from build123d import *

# Parameters (mm, degrees)
F1_DEPTH = 63.5
F2_DEPTH = 63.5


with BuildPart() as f1:
    # F0 (on Front) → F1 (new body)
    with BuildSketch(Plane.XZ):
        Polygon((-177.549966, -85.353864), (-177.549966, -100.162064), (-156.467966, -100.162064), (-13.263665, 3.495336), (-29.975966, 3.495336), (-51.057966, 3.495336), (-51.057966, -11.312864), (-72.139966, -11.312864), (-72.139966, -26.121064), (-93.221966, -26.121064), (-93.221966, -40.929264), (-114.303966, -40.929264), (-114.303966, -55.737464), (-135.385966, -55.737464), (-135.385966, -70.545664), (-156.467966, -70.545664), (-156.467966, -85.353864), align=None)
        Polygon((-29.975966, 3.495336), (-13.263665, 3.495336), (33.524034, 3.495336), (33.524034, 18.303536), (-29.975966, 18.303536), align=None)
    extrude(amount=F1_DEPTH)

    # F0 (on Front) → F2 (join)
    with BuildSketch(Plane.XZ):
        Polygon((-156.467966, 93.080176), (-29.975966, 3.495336), (-29.975966, 18.303536), (-29.975966, 33.111736), (-51.057966, 33.111736), (-51.057966, 47.919936), (-72.139966, 47.919936), (-72.139966, 62.728136), (-93.221966, 62.728136), (-93.221966, 77.536336), (-114.303966, 77.536336), (-114.303966, 92.344536), (-135.385966, 92.344536), (-135.385966, 107.152736), (-156.467966, 107.152736), align=None)
        Polygon((-29.975966, 3.495336), (-13.263665, 3.495336), (33.524034, 3.495336), (33.524034, 18.303536), (-29.975966, 18.303536), align=None)
    extrude(amount=-F2_DEPTH)


solid = f1.part
For this review, take the finished solid that the model builds, in its own axes (mm). A direction names the side the tool comes from. Round coordinates to 2 decimals unless told otherwise and drop trailing zeros. Loops run counter-clockwise (first coordinate to the right, second up) from the corner with the lowest first, then second, coordinate; pieces in that order, holes last. Notation, with made-up numbers: (43, 75) - (90, 75) arc R28 ccw to (90, 103) - close; hole circle Ø8 at (13, -30). An arc over 180 degrees is marked (long way). Put each result on its own line as item: value. Start each with the question number.
1. Consider section B-B on x = -62. State the section outline as (y, z) points, plus the area to 3 significant figures.
2. Insertion check: P1, Ø6.5, axis at x = -146.5, y = -27, coming from the +Z side; P2, Ø23, axis at x = -62, y = 37, coming from the +Z side; P3, Ø12, axis at x = -80, y = 29, coming from the -Z side. Each pin has a flat end and moves straight along its axis. Give the tip position at first contact, or say it passes through.
3. Consider section D-D on x = -8. State the section outline as (y, z) points.
4. Consider section A-A on y = -28. State the section outline as (x, z) points, plus the area to 3 significant figures.
5. For faces 1 (the flat face through (-29.976, 31, 26)), 2 (the flat face through (-146, -31, -70.546)), 3 (the flat face through (-29.976, -31, 11)), 4 (the flat face through (-102, 0, -48)), list the 3-axis set-ups (+Z, -Z, +X, -X, +Y, -Y) from which the entire face can be reached by the end or side of a thin tool; tool diameter is ignored.
6. For probe 1 along Z at (x, y) = (-11, 17.5); probe 2 along Y at (x, z) = (-95, 70); probe 3 along X at (y, z) = (-23, -54.5), list the stretches that pass through material, from the lowest coordinate up. Write a range as [from, to].
7. Consider section C-C on y = 27. State the section outline as (x, z) points.
Result sheet:
1. outline: (-63.5, -31.78) - (0, -31.78) - (0, -11.31) - (-63.5, -11.31) - close; (0, 26.18) - (63.5, 26.18) - (63.5, 47.92) - (0, 47.92) - close
1. area: 2,680 mm^2
2. P1: z = -70.55
2. P2: z = 62.73
2. P3: z = 34.67
3. outline: (-63.5, 3.5) - (63.5, 3.5) - (63.5, 18.3) - (-63.5, 18.3) - close
4. outline: (-177.55, -100.16) - (-156.47, -100.16) - (-13.26, 3.5) - (33.52, 3.5) - (33.52, 18.3) - (-29.98, 18.3) - (-29.98, 3.5) - (-51.06, 3.5) - (-51.06, -11.31) - (-72.14, -11.31) - (-72.14, -26.12) - (-93.22, -26.12) - (-93.22, -40.93) - (-114.3, -40.93) - (-114.3, -55.74) - (-135.39, -55.74) - (-135.39, -70.55) - (-156.47, -70.55) - (-156.47, -85.35) - (-177.55, -85.35) - close
4. area: 3,990 mm^2
5. face 1: +Z, +X, +Y, -Y
5. face 2: +Z, -X, +Y, -Y
5. face 3: +Z, -X, -Y
5. face 4: -Z, +X, -X, +Y
6. probe 1: [3.5, 18.3]
6. probe 2: [0, 63.5]
6. probe 3: [-114.3, -93.39]
7. outline: (-156.47, 93.08) - (-29.98, 3.5) - (33.52, 3.5) - (33.52, 18.3) - (-29.98, 18.3) - (-29.98, 33.11) - (-51.06, 33.11) - (-51.06, 47.92) - (-72.14, 47.92) - (-72.14, 62.73) - (-93.22, 62.73) - (-93.22, 77.54) - (-114.3, 77.54) - (-114.3, 92.34) - (-135.39, 92.34) - (-135.39, 107.15) - (-156.47, 107.15) - close
